Work out the finished part from the listing and answer in its coordinate system (mm). A direction names the side the tool comes from. Coordinates: 2 decimals unless noted, no trailing zeros. Order: outer loops, then holes, each group sorted by start corner. A loop starts at its lowest first (then second) coordinate and runs counter-clockwise, first axis right, second up. Notation, with made-up numbers: M -28,34 L 24,34 A24 cw 24,57 Z; hole C -17.5,69.5 d11. An arc over 180 degrees is marked long. Write item = value, one per line. Start each with the question number.
Q1. Find section D-D on z = 16. Give the vertices of the cut face in (x, y).
Q2. Determine the mould class of faces 1 (the flat face through (-4, -8, 17)), 2 (the flat face through (1, -8, 17)), 3 (the flat face through (-2, -7, 31)) for opening direction X: released by +X, released by -X, zero draft, split by the parting line, or undercut.
Q3. Each of these flat-tipped pins is pushed along its axis until it touches: P1, Ø6.5, axis at y = -6.5, z = 12, coming from the -X side; P2, Ø6, axis at x = -1, z = 24, coming from the +Y side; P3, Ø1.5, axis at x = -1.5, y = -3.5, coming from the +Z side. Where does it stop, or does it pass through?
Q4. A tool of negligible diameter and unlimited length cuts with its end or side. For faces 4 (the flat face through (-1, -8, 17)), 5 (the flat face through (4, -8, 17)), 6 (the flat face through (3, -7, 31)), 7 (the flat face through (1, -12, 44)), from which of +Z, -Z, +X, -X, +Y, -Y can it reach the whole face along a straight path? Write none if from no direction.
Q5. Find section C-C on z = 40.5. Give the vertices of the cut face in (x, y), and give its area (3 significant figures).
Q6. Find section B-B on y = 1.75. Give the vertices of the cut face in (x, z), and give its area (3 significant figures).
Q7. Straight lines are drawn through the part: line 1 along X through (y, z) = (-10, 28.5); line 2 along Y through (x, z) = (0, 5.75); line 3 along X through (y, z) = (0.5, 12.5). For each, find the intervals that lie inside material, in ascending order.
Q8. Find section A-A on x = 0. Give the vertices of the cut face in (y, z).
```python
from build123d import *

# Parameters (mm, degrees)
F1_DEPTH = 15
F2_DEPTH = 15
F3_DEPTH = 44
F4_R     = 4


with BuildPart() as f1:
    # F0 (on Top) → F1 (new body)
    with BuildSketch(Plane.XY):
        with BuildLine():
            ThreePointArc((4, -3), (4.7434164903, -1.5811388301), (5, 0))
            ThreePointArc((5, 0), (-1.5811388301, 4.7434164903), (-4, -3))
            ThreePointArc((-4, -3), (-2.6742346142, -4.2247448714), (-1, -4.8989794856))
            Line((-1, -4.8989794856), (-1, -3.8729833462))
            ThreePointArc((-1, -3.8729833462), (-2.4494897428, 3.1622776602), (4, 0))
            ThreePointArc((4, 0), (3.1622776602, -2.4494897428), (1, -3.8729833462))
            Line((1, -3.8729833462), (1, -4.8989794856))
            ThreePointArc((1, -4.8989794856), (2.6742346142, -4.2247448714), (4, -3))
        make_face()
    extrude(amount=F1_DEPTH)

    # F0 (on Top) → F2 (join)
    with BuildSketch(Plane.XY):
        with BuildLine():
            Line((-1, -7), (-4, -7))
            Line((-4, -7), (-4, -11))
            ThreePointArc((-4, -11), (-3.1622776602, -8.5505102572), (-1, -7.1270166538))
            Line((-1, -7.1270166538), (-1, -7))
        make_face()
        with BuildLine():
            Line((4, -11), (4, -7))
            Line((4, -7), (1, -7))
            Line((1, -7), (1, -7.1270166538))
            ThreePointArc((1, -7.1270166538), (3.1622776602, -8.5505102572), (4, -11))
        make_face()
        with BuildLine():
            ThreePointArc((-1, -7.1270166538), (-3.1622776602, -8.5505102572), (-4, -11))
            ThreePointArc((-4, -11), (0, -15), (4, -11))
            ThreePointArc((4, -11), (3.1622776602, -8.5505102572), (1, -7.1270166538))
            Line((1, -7.1270166538), (1, -11))
            ThreePointArc((1, -11), (0, -12), (-1, -11))
            Line((-1, -11), (-1, -7.1270166538))
        make_face()
        with BuildLine():
            ThreePointArc((-1, -4.8989794856), (-2.6742346142, -4.2247448714), (-4, -3))
            Line((-4, -3), (-4, -7))
            Line((-4, -7), (-1, -7))
            Line((-1, -7), (-1, -4.8989794856))
        make_face()
        with BuildLine():
            Line((4, -7), (4, -3))
            ThreePointArc((4, -3), (2.6742346142, -4.2247448714), (1, -4.8989794856))
            Line((1, -4.8989794856), (1, -7))
            Line((1, -7), (4, -7))
        make_face()
    extrude(amount=F2_DEPTH)

    # F0 (on Top) → F3 (join)
    with BuildSketch(Plane.XY):
        with BuildLine():
            ThreePointArc((-1, -7.1270166538), (-3.1622776602, -8.5505102572), (-4, -11))
            ThreePointArc((-4, -11), (0, -15), (4, -11))
            ThreePointArc((4, -11), (3.1622776602, -8.5505102572), (1, -7.1270166538))
            Line((1, -7.1270166538), (1, -11))
            ThreePointArc((1, -11), (0, -12), (-1, -11))
            Line((-1, -11), (-1, -7.1270166538))
        make_face()
        with BuildLine():
            Line((-1, -7), (-4, -7))
            Line((-4, -7), (-4, -11))
            ThreePointArc((-4, -11), (-3.1622776602, -8.5505102572), (-1, -7.1270166538))
            Line((-1, -7.1270166538), (-1, -7))
        make_face()
        with BuildLine():
            Line((4, -11), (4, -7))
            Line((4, -7), (1, -7))
            Line((1, -7), (1, -7.1270166538))
            ThreePointArc((1, -7.1270166538), (3.1622776602, -8.5505102572), (4, -11))
        make_face()
    extrude(amount=F3_DEPTH)

    # F4
    f4_edges = [f1.edges().sort_by_distance(p)[0] for p in [
        (-2.5, -7, 15),
        (2.5, -7, 15),
    ]]
    fillet(f4_edges, radius=F4_R)


solid = f1.part
```
Findings below:
q1.outline = M -4,-11 A4 ccw 4,-11 L 4,-5.65 L 1,-5.65 L 1,-11 A1 cw -1,-11 L -1,-5.65 L -4,-5.65 Z
q2.face_1 = released by -X
q2.face_2 = undercut
q2.face_3 = zero draft
q3.P1 = -4
q3.P2 = -7
q3.P3 = 15.2
q4.face_4 = +Z, -Z
q4.face_5 = +Z, -Z, +X, -Y
q4.face_6 = +Z, +X, -X, +Y
q4.face_7 = +Z, +X, -X, +Y, -Y
q5.outline = M -4,-11 A4 ccw 4,-11 L 4,-7 L 1,-7 L 1,-11 A1 cw -1,-11 L -1,-7 L -4,-7 Z
q5.area = 47.6 mm^2
q6.outline = M -4.68,0 L -3.6,0 L -3.6,15 L -4.68,15 Z; M 3.6,0 L 4.68,0 L 4.68,15 L 3.6,15 Z
q6.area = 32.6 mm^2
q7.line_1 = -4 to -1, 1 to 4
q7.line_2 = -15 to -12, 4 to 5
q7.line_3 = -4.97 to -3.97, 3.97 to 4.97
q8.outline = M -15,0 L -12,0 L -12,44 L -15,44 Z; M 4,0 L 5,0 L 5,15 L 4,15 Z
